```python
from build123d import *

# Parameters (mm, degrees)
BOSS_EXTRUDE1_DEPTH = 6.35


with BuildPart() as part:
    # Sketch1 → Boss-Extrude1 (new body)
    with BuildSketch(Plane.XY):
        with BuildLine():
            Line((-10, 35), (-10, 0))
            Line((-10, 0), (10, 0))
            Line((10, 0), (10, 35))
            ThreePointArc((10, 35), (0, 45), (-10, 35))
        make_face()
        with BuildLine():
            Line((3, 35), (3, 10))
            ThreePointArc((3, 10), (0, 7), (-3, 10))
            Line((-3, 10), (-3, 35))
            ThreePointArc((-3, 35), (0, 38), (3, 35))
        make_face(mode=Mode.SUBTRACT)
    extrude(amount=BOSS_EXTRUDE1_DEPTH)


solid = part.part
```
Part model, mm, in its own coordinate system. A direction names the side the tool comes from. Give positions to 0.01 mm unless a question says otherwise; leave off trailing zeros. Loops run counter-clockwise (first coordinate to the right, second up) from the corner with the lowest first, then second, coordinate; pieces in that order, holes last. Notation, with made-up numbers: M 87,37.25 L 99,37.25 A17 ccw 99,51.25 Z; hole C 26.25,-11.75 d11. An arc over 180 degrees is marked long. Return JSON: item names as keys, results as strings.
1) Saw through at C-C, the plane z = 2.75. List the corners of the cut face in (x, y), then the cut area to 3 significant figures.
Calculated:
{"outline": "M -10,0 L 10,0 L 10,35 A10 ccw -10,35 Z; hole M -3,10 A3 ccw 3,10 L 3,35 A3 ccw -3,35 Z", "area": "679 mm2"}
2) Drill centre lines: line 1 (X direction, y = 20.5, z = 2.5); line 2 (Y direction, x = -1.5, z = 1); line 3 (Y direction, x = -1, z = 5). Where is each one in solid material? Low to high.
Calculated:
{"line 1": "x = -10 to -3, 3 to 10", "line 2": "y = 0 to 7.4, 37.6 to 44.89", "line 3": "y = 0 to 7.17, 37.83 to 44.95"}
3) 3-axis set-ups, long thin cutter, end or side, ignore diameter. For faces 1 (the face through (-10, 18, 3)), 2 (the face through (0, 38, 3)): which of +Z, -Z, +X, -X, +Y, -Y reach the whole face in a straight line?
Calculated:
{"face 1": "+Z, -Z, -X, +Y, -Y", "face 2": "+Z, -Z"}
4) Pull direction Y, two halves, no side cores. Call faces 3 (the face through (0, 7, 3)), 4 (the face through (10, 17, 3)), 5 (the face through (0, 0, 3)): released by +Y, released by -Y, zero draft, split by the parting line, or undercut.
Calculated:
{"face 3": "undercut", "face 4": "zero draft", "face 5": "released by -Y"}
5) Saw through at D-D, the plane x = 6. List the corners of the cut face in (y, z).
Calculated:
{"outline": "M 0,0 L 43,0 L 43,6.35 L 0,6.35 Z"}
6) Saw through at B-B, the plane x = 0. List the corners of the cut face in (y, z), then the cut area to 3 significant figures.
Calculated:
{"outline": "M 0,0 L 7,0 L 7,6.35 L 0,6.35 Z; M 38,0 L 45,0 L 45,6.35 L 38,6.35 Z", "area": "88.9 mm2"}
7) Saw through at A-A, the plane y = 29. List the corners of the cut face in (x, z).
Calculated:
{"outline": "M -10,0 L -3,0 L -3,6.35 L -10,6.35 Z; M 3,0 L 10,0 L 10,6.35 L 3,6.35 Z"}
